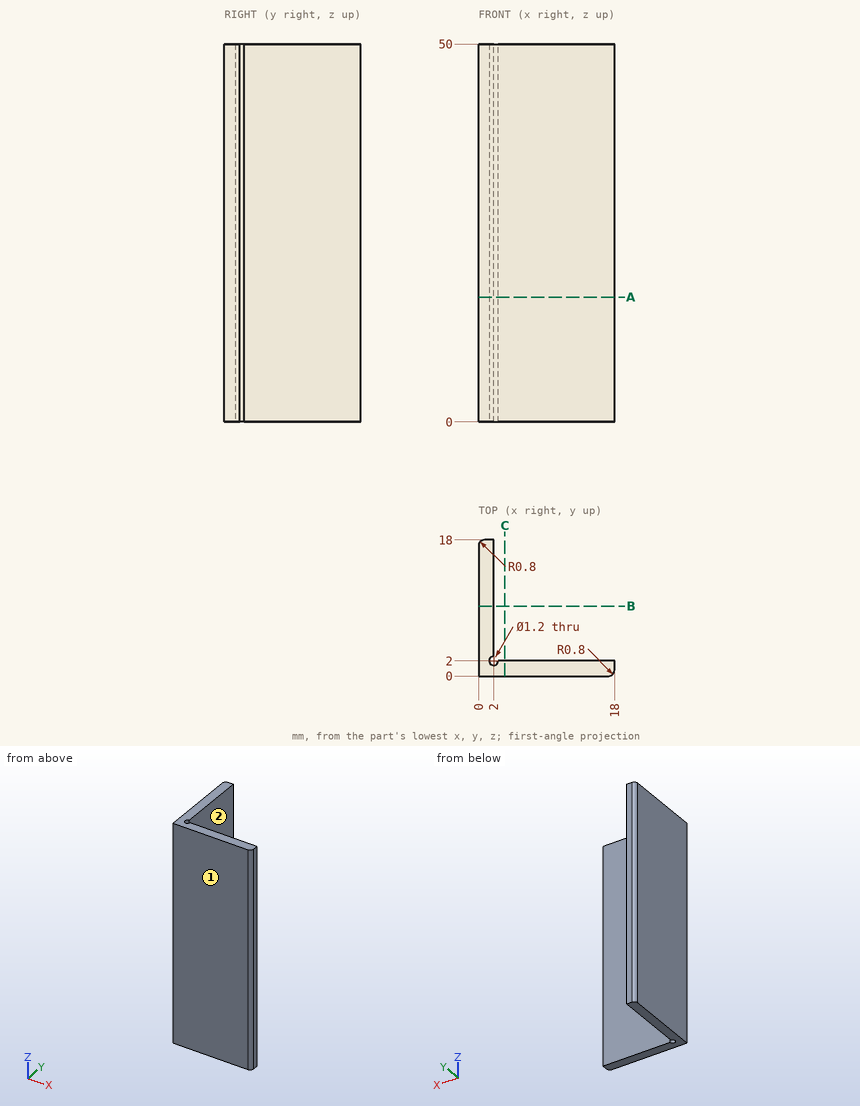
Can you work these out from the drawing? Everything is in mm from the part's minimum corner. A direction names the side the tool comes from. Round coordinates to 2 decimals unless told otherwise and drop trailing zeros. Order: outer loops, then holes, each group sorted by start corner. A loop starts at its lowest first (then second) coordinate and runs counter-clockwise, first axis right, second up. Notation, with made-up numbers: (-14.5, 5) -> (-10.5, 5) arc R12 ccw to (-10.5, 18) -> close; hole circle Ø10 at (11, 30.25). An arc over 180 degrees is marked (long way). Return JSON: item names as keys, results as strings. Group by question number.
1. Which directions (+Z, -Z, +X, -X, +Y, -Y) give clear straight access to the entire face, cutting with the end or side of a thin tool? Please do the marked faces 1 and 2.
2. Will this pin go through, and if not, where does the flat tip stop? pin 1 (7.5 mm diameter, centred on x = 9, z = 30.5, fed in from +Y).
3. If we section it at A-A, the plane z = 16.5: Write out the boundary of the cut face in (x, y).
4. I need wall thicknesses on line 1 (Y direction, x = 6.5, z = 19). Which ranges of the line are inside material? Lowest first, please. Write a range as [from, to].
5. If we section it at B-B, the plane y = 9.25: Write out the boundary of the cut face in (x, z).
Output values:
{
 "1": {"face 1": "+Z, -Z, +X, -X, -Y", "face 2": "+Z, -Z, +X, +Y"},
 "2": {"pin 1": "y = 2"},
 "3": {"outline": "(0, 0) -> (17.2, 0) arc R0.8 ccw to (18, 0.8) -> (18, 2) -> (2.6, 2) arc R0.6 cw (long way) to (2, 2.6) -> (2, 18) -> (0.8, 18) arc R0.8 ccw to (0, 17.2) -> close"},
 "4": {"line 1": "[0, 2]"},
 "5": {"outline": "(0, 0) -> (2, 0) -> (2, 50) -> (0, 50) -> close"}
}
